Check sheet for the modelled part. Datum: model origin and axes. Units: mm. Face numbers are marked on the shaded views. A direction names the side the tool comes from. Coordinates: 2 decimals unless noted, no trailing zeros. Order: outer loops, then holes, each group sorted by start corner. A loop starts at its lowest first (then second) coordinate and runs counter-clockwise, first axis right, second up.
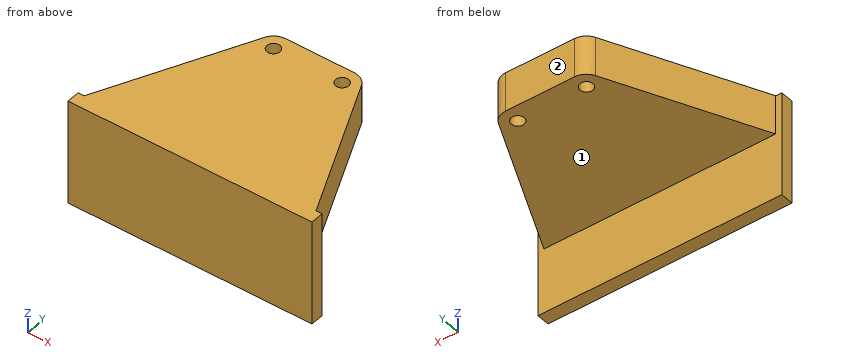
from build123d import *

# Parameters (mm, degrees)
SKETCH1_R           = 1.5875
BOSS_EXTRUDE1_DEPTH = 9.525
SKETCH2_W           = 59.519961842
SKETCH2_H           = 3.175
BOSS_EXTRUDE2_DEPTH = 25.4


with BuildPart() as part:
    # Sketch1 → Boss-Extrude1 (new body)
    with BuildSketch(Plane.XY):
        with BuildLine():
            Line((0, 0), (17.924948252, 38.440175577))
            ThreePointArc((17.924948252, 38.440175577), (19.330869413, 40.043321409), (21.377980921, 40.64))
            Line((21.377980921, 40.64), (38.141980921, 40.64))
            ThreePointArc((38.141980921, 40.64), (40.189092429, 40.043321409), (41.59501359, 38.440175577))
            Line((41.59501359, 38.440175577), (59.519961842, 0))
            Line((59.519961842, 0), (0, 0))
        make_face()
        with Locations((21.377980921, 36.83)):
            Circle(SKETCH1_R, mode=Mode.SUBTRACT)
        with Locations((38.141980921, 36.83)):
            Circle(SKETCH1_R, mode=Mode.SUBTRACT)
    extrude(amount=BOSS_EXTRUDE1_DEPTH)

    # Sketch2 → Boss-Extrude2 (add)
    with BuildSketch(Plane.XY.offset(9.525)):
        with Locations((29.759980921, 1.5875)):
            Rectangle(SKETCH2_W, SKETCH2_H)
    extrude(amount=-BOSS_EXTRUDE2_DEPTH)


solid = part.part
(1) Cross-section at B-B (y = 36.83). Enter the section's corners in (x, z) (3 decimals), and give its area (3 significant figures).
Filled in:
outline: (17.174, 0) - (19.79, 0) - (19.79, 9.525) - (17.174, 9.525) - close; (22.965, 0) - (36.554, 0) - (36.554, 9.525) - (22.965, 9.525) - close; (39.729, 0) - (42.346, 0) - (42.346, 9.525) - (39.729, 9.525) - close
area: 179 mm2
(2) Cross-section at A-A (z = 1.75). Enter the section's corners in (x, y) (1 decimal).
Filled in:
outline: (0, 0) - (59.5, 0) - (59.5, 3.2) - (58, 3.2) - (41.6, 38.4) arc R3.8 ccw to (38.1, 40.6) - (21.4, 40.6) arc R3.8 ccw to (17.9, 38.4) - (1.5, 3.2) - (0, 3.2) - close; hole circle Ø3.2 at (21.4, 36.8); hole circle Ø3.2 at (38.1, 36.8)
(3) Cross-section at D-D (z = -9). Enter the section's corners in (x, y) (3 decimals).
Filled in:
outline: (0, 0) - (59.52, 0) - (59.52, 3.175) - (0, 3.175) - close
(4) Thickness scan on probe 1 along Y at (x, z) = (20, -6) (3 decimals); probe 2 along Z at (x, y) = (8, 11) (3 decimals); probe 3 along Y at (x, z) = (21.5, 8.25). Record the ranges inside material, lowest first.
Filled in:
probe 1: y = 0 to 3.175
probe 2: z = 0 to 9.525
probe 3: y = 0 to 35.25, 38.41 to 40.64
(5) Tool access check on the marked faces 1 and 2. Record the directions out of +Z, -Z, +X, -X, +Y, -Y that give a thin tool (end or side, any length) a straight path to the whole face; none if there is none.
Filled in:
face 1: -Z, +X, -X, +Y
face 2: +Z, -Z, +X, -X, +Y
(6) Go/stop test with flat-tipped pins: P1, Ø1, axis at x = 42.5, z = -10.5, coming from the +Y side (3 decimals); P2, Ø1.5, axis at y = 4.5, z = 0, coming from the +X side; P3, Ø12, axis at y = 27.5, z = 7, coming from the -X side. Record where each tip stops, or that it passes through.
Filled in:
P1: stops at y = 3.175
P2: stops at x = 57.77
P3: stops at x = 10.03
(7) Cross-section at C-C (x = 6). Enter the section's corners in (y, z) (3 decimals).
Filled in:
outline: (0, -15.875) - (3.175, -15.875) - (3.175, 0) - (12.867, 0) - (12.867, 9.525) - (0, 9.525) - close
